Input: dimensioned drawing with shaded views. Units: mm. Origin: part minimum x, y, z. Round coordinates to 2 decimals unless told otherwise and drop trailing zeros. Loops run counter-clockwise (first coordinate to the right, second up) from the corner with the lowest first, then second, coordinate; pieces in that order, holes last. Notation, with made-up numbers: M 34,-6 L 88,-6 A32 ccw 88,26 Z; hole C 73.5,34 d10. An arc over 180 degrees is marked long. Answer as CSV lines item,"result". Start each with the question number.
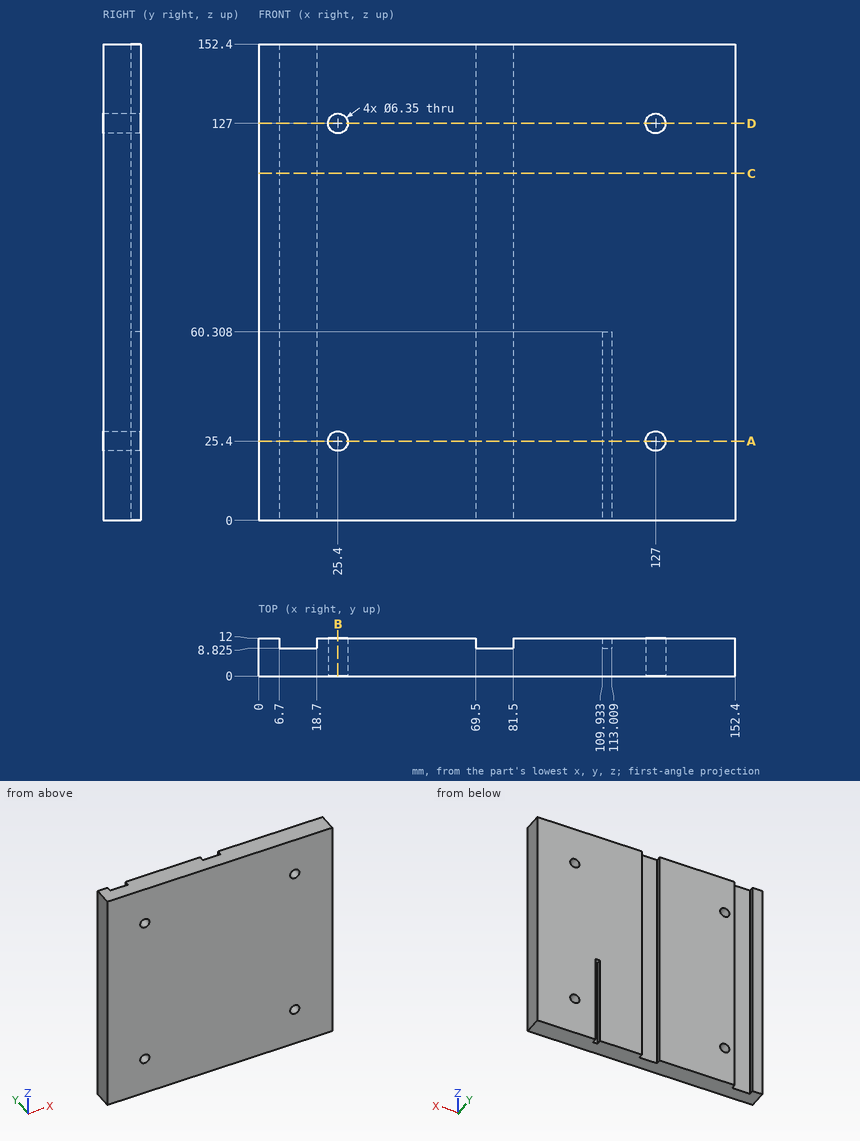
1) Section C-C, the plane z = 111. Return loops of the section in (x, y) (1 decimal).
2) Section B-B, the plane x = 25.4. Return loops of the section in (y, z) (1 decimal), and give its area (3 significant figures).
3) Section A-A, the plane z = 25.4. Return loops of the section in (x, y) (1 decimal).
4) Ray query, line 1 along X through (y, z) = (3, 126.5) (1 decimal); line 2 along X through (y, z) = (10.25, 46); line 3 along X through (y, z) = (2.5, 25.4) (1 decimal). Return the intervals inside material, ascending.
5) Section D-D, the plane z = 127. Return loops of the section in (x, y) (1 decimal).
6) Contact query for flat-ended pins moving along their axis: pin 1 Ø1.6 at (y, z) = (10.5, 92) entering from -X; pin 2 Ø1.5 at (x, z) = (111, 36.5) entering from +Y (1 decimal); pin 3 Ø5.5 at (x, z) = (25.4, 25.4) entering from +Y. Output: stop coordinate, or through.
Findings below:
1,outline,"M 0,0 L 152.4,0 L 152.4,12 L 81.5,12 L 81.5,8.8 L 69.5,8.8 L 69.5,12 L 18.7,12 L 18.7,8.8 L 6.7,8.8 L 6.7,12 L 0,12 Z"
2,outline,"M 0,0 L 12,0 L 12,22.2 L 0,22.2 Z; M 0,28.6 L 12,28.6 L 12,123.8 L 0,123.8 Z; M 0,130.2 L 12,130.2 L 12,152.4 L 0,152.4 Z"
2,area,"1,680 mm²"
3,outline,"M 0,0 L 22.2,0 L 22.2,12 L 18.7,12 L 18.7,8.8 L 6.7,8.8 L 6.7,12 L 0,12 Z; M 28.6,0 L 123.8,0 L 123.8,12 L 113,12 L 113,8.8 L 109.9,8.8 L 109.9,12 L 81.5,12 L 81.5,8.8 L 69.5,8.8 L 69.5,12 L 28.6,12 Z; M 130.2,0 L 152.4,0 L 152.4,12 L 130.2,12 Z"
4,line 1,"0 to 22.3, 28.5 to 123.9, 130.1 to 152.4"
4,line 2,"0 to 6.7, 18.7 to 69.5, 81.5 to 109.93, 113.01 to 152.4"
4,line 3,"0 to 22.2, 28.6 to 123.8, 130.2 to 152.4"
5,outline,"M 0,0 L 22.2,0 L 22.2,12 L 18.7,12 L 18.7,8.8 L 6.7,8.8 L 6.7,12 L 0,12 Z; M 28.6,0 L 123.8,0 L 123.8,12 L 81.5,12 L 81.5,8.8 L 69.5,8.8 L 69.5,12 L 28.6,12 Z; M 130.2,0 L 152.4,0 L 152.4,12 L 130.2,12 Z"
6,pin 1,"x = 0"
6,pin 2,"y = 8.8"
6,pin 3,"through"
